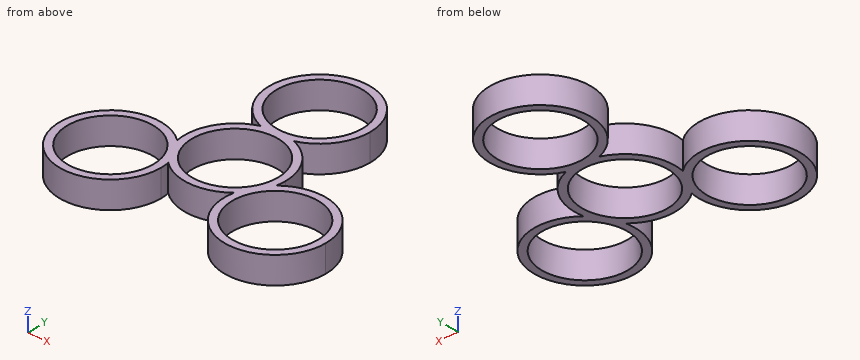
```python
from build123d import *

# Parameters (mm, degrees)
F0_R     = 11.2
F1_DEPTH = 7


with BuildPart() as f1:
    # F0 (on Top) → F1 (new body)
    with BuildSketch(Plane.XY):
        with BuildLine():
            ThreePointArc((12.968803749, -2.4597010632), (13.1420738372, -1.2352713292), (13.2, 0))
            ThreePointArc((13.2, 0), (10.7637341369, 7.6408132702), (4.3542382681, 12.4611640349))
            ThreePointArc((4.3542382681, 12.4611640349), (0, 11.7223280698), (-4.3542382681, 12.4611640349))
            ThreePointArc((-4.3542382681, 12.4611640349), (-11.43153533, 6.6), (-12.968803749, -2.4597010632))
            ThreePointArc((-12.968803749, -2.4597010632), (-10.1518338999, -5.8611640349), (-8.6145654809, -10.0014629717))
            ThreePointArc((-8.6145654809, -10.0014629717), (0, -13.2), (8.6145654809, -10.0014629717))
            ThreePointArc((8.6145654809, -10.0014629717), (10.1518338999, -5.8611640349), (12.968803749, -2.4597010632))
        make_face()
        Circle(F0_R, mode=Mode.SUBTRACT)
        with BuildLine():
            ThreePointArc((-4.3542382681, 12.4611640349), (0, 11.7223280698), (4.3542382681, 12.4611640349))
            ThreePointArc((4.3542382681, 12.4611640349), (0, 13.2), (-4.3542382681, 12.4611640349))
        make_face()
        with BuildLine():
            ThreePointArc((-4.3542382681, 12.4611640349), (0, 13.2), (4.3542382681, 12.4611640349))
            ThreePointArc((4.3542382681, 12.4611640349), (10.7637341369, 17.2815147996), (13.2, 24.9223280698))
            ThreePointArc((13.2, 24.9223280698), (-7.6408132702, 35.6860622067), (-4.3542382681, 12.4611640349))
        make_face()
        with Locations((0, 24.9223280698)):
            Circle(F0_R, mode=Mode.SUBTRACT)
        with BuildLine():
            ThreePointArc((34.7833692299, -12.4611640349), (27.0846297969, -0.4621585689), (12.968803749, -2.4597010632))
            ThreePointArc((12.968803749, -2.4597010632), (11.43153533, -6.6), (8.6145654809, -10.0014629717))
            ThreePointArc((8.6145654809, -10.0014629717), (20.3480979007, -25.6032378721), (34.7833692299, -12.4611640349))
        make_face()
        with Locations((21.5833692299, -12.4611640349)):
            Circle(F0_R, mode=Mode.SUBTRACT)
        with BuildLine():
            ThreePointArc((8.6145654809, -10.0014629717), (11.43153533, -6.6), (12.968803749, -2.4597010632))
            ThreePointArc((12.968803749, -2.4597010632), (10.1518338999, -5.8611640349), (8.6145654809, -10.0014629717))
        make_face()
        with BuildLine():
            ThreePointArc((-8.6145654809, -10.0014629717), (-10.1518338999, -5.8611640349), (-12.968803749, -2.4597010632))
            ThreePointArc((-12.968803749, -2.4597010632), (-11.43153533, -6.6), (-8.6145654809, -10.0014629717))
        make_face()
        with BuildLine():
            ThreePointArc((-8.6145654809, -10.0014629717), (-11.43153533, -6.6), (-12.968803749, -2.4597010632))
            ThreePointArc((-12.968803749, -2.4597010632), (-33.5823746959, -17.9624246019), (-8.3833692299, -12.4611640349))
            ThreePointArc((-8.3833692299, -12.4611640349), (-8.4412953927, -11.2258927057), (-8.6145654809, -10.0014629717))
        make_face()
        with Locations((-21.5833692299, -12.4611640349)):
            Circle(F0_R, mode=Mode.SUBTRACT)
    extrude(amount=F1_DEPTH)


solid = f1.part
```
Work out the finished part from the listing and answer in its coordinate system (mm). Give positions to 0.01 mm unless a question says otherwise; leave off trailing zeros. Loops run counter-clockwise (first coordinate to the right, second up) from the corner with the lowest first, then second, coordinate; pieces in that order, holes last. Notation, with made-up numbers: (4, 21.25) - (58, 21.25) arc R26 cw to (58, 45.25) - close; hole circle Ø8 at (28.5, -28). An arc over 180 degrees is marked (long way). One line per question, with ' | ' between items.
(1) The part is cut by section A-A (x = 0). Write down the section's boundary in (y, z).
Recorded:
outline: (-13.2, 0) - (-11.2, 0) - (-11.2, 7) - (-13.2, 7) - close; (11.2, 0) - (13.72, 0) - (13.72, 7) - (11.2, 7) - close; (36.12, 0) - (38.12, 0) - (38.12, 7) - (36.12, 7) - close
(2) The part is cut by section C-C (y = -14). Write down the section's boundary in (x, z).
Recorded:
outline: (-34.69, 0) - (-32.68, 0) - (-32.68, 7) - (-34.69, 7) - close; (-10.49, 0) - (-8.47, 0) - (-8.47, 7) - (-10.49, 7) - close; (8.47, 0) - (10.49, 0) - (10.49, 7) - (8.47, 7) - close; (32.68, 0) - (34.69, 0) - (34.69, 7) - (32.68, 7) - close
(3) Straight lines are drawn through the part: probe 1 along Y at (x, z) = (-0.5, 4.5); probe 2 along X at (y, z) = (-4, 4.25); probe 3 along Y at (x, z) = (-3, 5.5). For each, find the intervals that lie inside material, in ascending order.
Recorded:
probe 1: y = -13.19 to -11.19, 11.19 to 13.73, 36.11 to 38.11 | probe 2: x = -31.71 to -28.92, -14.25 to -10.46, 10.46 to 14.25, 28.92 to 31.71 | probe 3: y = -12.85 to -10.79, 10.79 to 14.13, 35.71 to 37.78
(4) Each of these flat-tipped pins is pushed along its axis until it touches: pin 1 Ø1 at (x, z) = (23, 4.5) entering from -Y; pin 2 Ø1.5 at (y, z) = (-17, 1) entering from -X; pin 3 Ø2 at (y, z) = (26.5, 4) entering from -X. Where does it stop, or does it pass through?
Recorded:
pin 1: stops at y = -25.63 | pin 2: stops at x = -34.23 | pin 3: stops at x = -13.19
(5) The part is cut by section B-B (y = 19.5). Write down the section's boundary in (x, z), then the cut area to 3 significant figures.
Recorded:
outline: (-12.03, 0) - (-9.8, 0) - (-9.8, 7) - (-12.03, 7) - close; (9.8, 0) - (12.03, 0) - (12.03, 7) - (9.8, 7) - close | area: 31.3 mm²
(6) The part is cut by section D-D (x = -24). Write down the section's boundary in (y, z) (3 decimals), then the cut area to 3 significant figures.
Recorded:
outline: (-25.438, 0) - (-23.397, 0) - (-23.397, 7) - (-25.438, 7) - close; (-1.525, 0) - (0.516, 0) - (0.516, 7) - (-1.525, 7) - close | area: 28.6 mm²
